from build123d import *

# Parameters (mm, degrees)
SKETCH1_W           = 138.92560988
SKETCH1_H           = 12.7
SKETCH1_R           = 1.778
BOSS_EXTRUDE1_DEPTH = 3.175
SKETCH2_W           = 3.175
SKETCH2_H           = 12.7
BOSS_EXTRUDE2_DEPTH = 63.5
SKETCH3_R           = 1.778
CUT_EXTRUDE1_DEPTH  = 152.4


with BuildPart() as part:
    # Sketch1 → Boss-Extrude1 (new body)
    with BuildSketch(Plane.XY):
        with Locations((-69.46280494, -6.35)):
            Rectangle(SKETCH1_W, SKETCH1_H)
        with Locations((-94.86280494, -6.35)):
            Circle(SKETCH1_R, mode=Mode.SUBTRACT)
        with Locations((-44.06280494, -6.35)):
            Circle(SKETCH1_R, mode=Mode.SUBTRACT)
    extrude(amount=BOSS_EXTRUDE1_DEPTH)

    # Sketch2 → Boss-Extrude2 (add)
    with BuildSketch(Plane.XY.offset(3.175)):
        with Locations((-137.33810988, -6.35)):
            Rectangle(SKETCH2_W, SKETCH2_H)
        with Locations((-1.5875, -6.35)):
            Rectangle(SKETCH2_W, SKETCH2_H)
    extrude(amount=BOSS_EXTRUDE2_DEPTH)

    # Sketch3 → Cut-Extrude1 (cut)
    with BuildSketch(Plane(origin=(0, 0, 0), x_dir=(0, 0, -1), z_dir=(1, 0, 0))):
        with Locations((-56.840236332, -6.35)):
            Circle(SKETCH3_R)
    extrude(amount=-CUT_EXTRUDE1_DEPTH, mode=Mode.SUBTRACT)


solid = part.part
Source: CAD feature listing. Evaluate the final solid. Frame: model axes, mm. A direction names the side the tool comes from. Give positions to 0.01 mm unless a question says otherwise; leave off trailing zeros. Loops run counter-clockwise (first coordinate to the right, second up) from the corner with the lowest first, then second, coordinate; pieces in that order, holes last. Notation, with made-up numbers: (79.5, 16) -> (112.5, 16) arc R23 ccw to (112.5, 36) -> close; hole circle Ø5 at (65.5, 12.5). An arc over 180 degrees is marked (long way). Use a Markdown table: item, result. Add a question column.
1) First-contact query: pin 1 (3 mm diameter, centred on y = -6.35, z = 56.84, fed in from -X). Flat tip, straight axial feed; report the tip coordinate or a pass-through.
2) Section query B-B, the plane y = -6.35. Return the cut outline in (x, z) (3 decimals), then the cut area to 3 significant figures.
3) Section query C-C, the plane z = 56.5. Return the cut outline in (x, y) (3 decimals), then the cut area to 3 significant figures.
4) Section query D-D, the plane x = -13. Return the cut outline in (y, z) (3 decimals), then the cut area to 3 significant figures.
5) Pull-direction query (Y, two-part tool) for faces 1 (the face through (-70, -12.7, 1)), 2 (the face through (0, -6, 33)), 3 (the face through (-45.5, -7.4, 1.6)); classes: +Y half, -Y half, draft (parallel to the pull), parting line (faces both ways), or undercut.
6) Section query A-A, the plane z = 9. Return the cut outline in (x, y) (3 decimals), then the cut area to 3 significant figures.
7) Line query: line 1 along X through (y, z) = (-5.75, 36) (3 decimals); line 2 along Z through (x, y) = (-132, -3.5) (3 decimals). Output: solid intervals per line, ascending. Write a range as [from, to].
8) Reachability of faces 4 (the face through (-70, -6, 3.175)), 5 (the face through (-137.316, -6.272, 58.617)) from +Z, -Z, +X, -X, +Y, -Y: full face, straight path, thin tool, end or side. Return the list, or none.
Numbers:
| question | item | result |
|---|---|---|
| 1 | pin 1 | passes through |
| 2 | outline | (-138.926, 0) -> (-96.641, 0) -> (-96.641, 3.175) -> (-135.751, 3.175) -> (-135.751, 55.062) -> (-138.926, 55.062) -> close; (-138.926, 58.618) -> (-135.751, 58.618) -> (-135.751, 66.675) -> (-138.926, 66.675) -> close; (-93.085, 0) -> (-45.841, 0) -> (-45.841, 3.175) -> (-93.085, 3.175) -> close; (-42.285, 0) -> (0, 0) -> (0, 55.062) -> (-3.175, 55.062) -> (-3.175, 3.175) -> (-42.285, 3.175) -> close; (-3.175, 58.618) -> (0, 58.618) -> (0, 66.675) -> (-3.175, 66.675) -> close |
| 2 | area | 799 mm2 |
| 3 | outline | (-138.926, -12.7) -> (-135.751, -12.7) -> (-135.751, -8.095) -> (-138.926, -8.095) -> close; (-138.926, -4.605) -> (-135.751, -4.605) -> (-135.751, 0) -> (-138.926, 0) -> close; (-3.175, -12.7) -> (0, -12.7) -> (0, -8.095) -> (-3.175, -8.095) -> close; (-3.175, -4.605) -> (0, -4.605) -> (0, 0) -> (-3.175, 0) -> close |
| 3 | area | 58.5 mm2 |
| 4 | outline | (-12.7, 0) -> (0, 0) -> (0, 3.175) -> (-12.7, 3.175) -> close |
| 4 | area | 40.3 mm2 |
| 5 | face 1 | -Y half |
| 5 | face 2 | draft |
| 5 | face 3 | undercut |
| 6 | outline | (-138.926, -12.7) -> (-135.751, -12.7) -> (-135.751, 0) -> (-138.926, 0) -> close; (-3.175, -12.7) -> (0, -12.7) -> (0, 0) -> (-3.175, 0) -> close |
| 6 | area | 80.6 mm2 |
| 7 | line 1 | x = [-138.926, -135.751], [-3.175, 0] |
| 7 | line 2 | z = [0, 3.175] |
| 8 | face 4 | +Z, +Y, -Y |
| 8 | face 5 | +X, -X |
